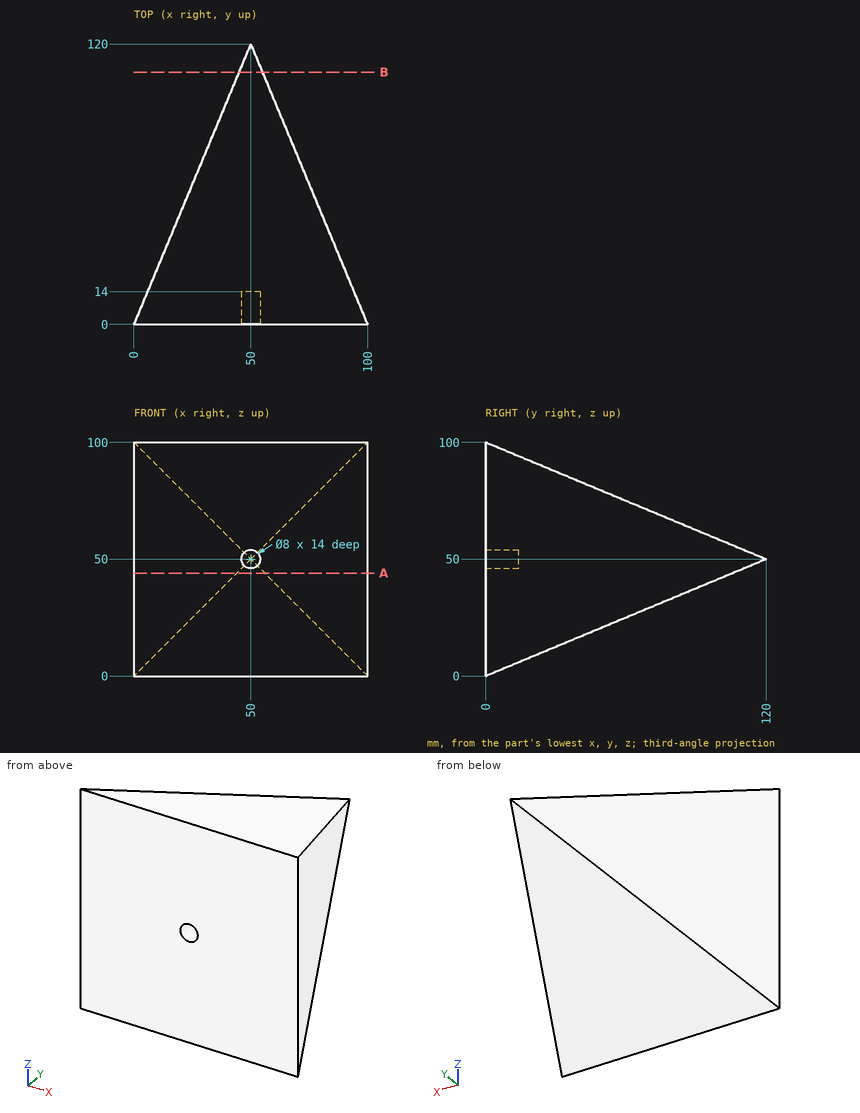
Study the drawing (mm; zero at the part's minimum x, y, z) and answer. Give positions to 0.01 mm unless a question says otherwise; leave off trailing zeros. Loops run counter-clockwise (first coordinate to the right, second up) from the corner with the lowest first, then second, coordinate; pieces in that order, holes last. Notation, with made-up numbers: (-13.5, -36) - (23.5, -36) arc R17 ccw to (23.5, -11) - close; hole circle Ø5 at (-12.75, 30.25). An arc over 180 degrees is marked (long way). One line per question, with ' | ' between items.
(1) Straight lines are drawn through the part: probe 1 along X at (y, z) = (8, 50); probe 2 along X at (y, z) = (11.25, 50); probe 3 along X at (y, z) = (41.5, 20.5). For each, find the intervals that lie inside material, in ascending order.
Recorded:
probe 1: x = 3.33 to 46, 54 to 96.67 | probe 2: x = 4.69 to 46, 54 to 95.31 | probe 3: x = 17.29 to 82.71
(2) Each of these flat-tipped pins is pushed along its axis until it touches: pin 1 Ø2 at (x, z) = (79.5, 64.5) entering from +Y; pin 2 Ø4 at (x, y) = (79, 44) entering from +Z; pin 3 Ø2 at (x, z) = (61.5, 76) entering from +Y. Where does it stop, or does it pass through?
Recorded:
pin 1: stops at y = 51.6 | pin 2: stops at z = 82.5 | pin 3: stops at y = 60
(3) The part is cut by section B-B (y = 108). Write down the section's boundary in (x, z), then the cut area to 3 significant figures.
Recorded:
outline: (45, 45) - (55, 45) - (55, 55) - (45, 55) - close | area: 100 mm²
(4) The part is cut by section A-A (z = 44). Write down the section's boundary in (x, y), then the cut area to 3 significant figures.
Recorded:
outline: (0, 0) - (100, 0) - (56, 105.6) - (44, 105.6) - close | area: 5,910 mm²
